Can you work these out from the drawing? Everything is in mm from the part's minimum corner. A direction names the side the tool comes from. Round coordinates to 2 decimals unless told otherwise and drop trailing zeros. Order: outer loops, then holes, each group sorted by start corner. A loop starts at its lowest first (then second) coordinate and runs counter-clockwise, first axis right, second up. Notation, with made-up numbers: (29.5, 46.25) -> (65.5, 46.25) arc R33 ccw to (65.5, 78.25) -> close; hole circle Ø7 at (33.5, 20). An arc over 180 degrees is marked (long way). One line per item, written item: value.
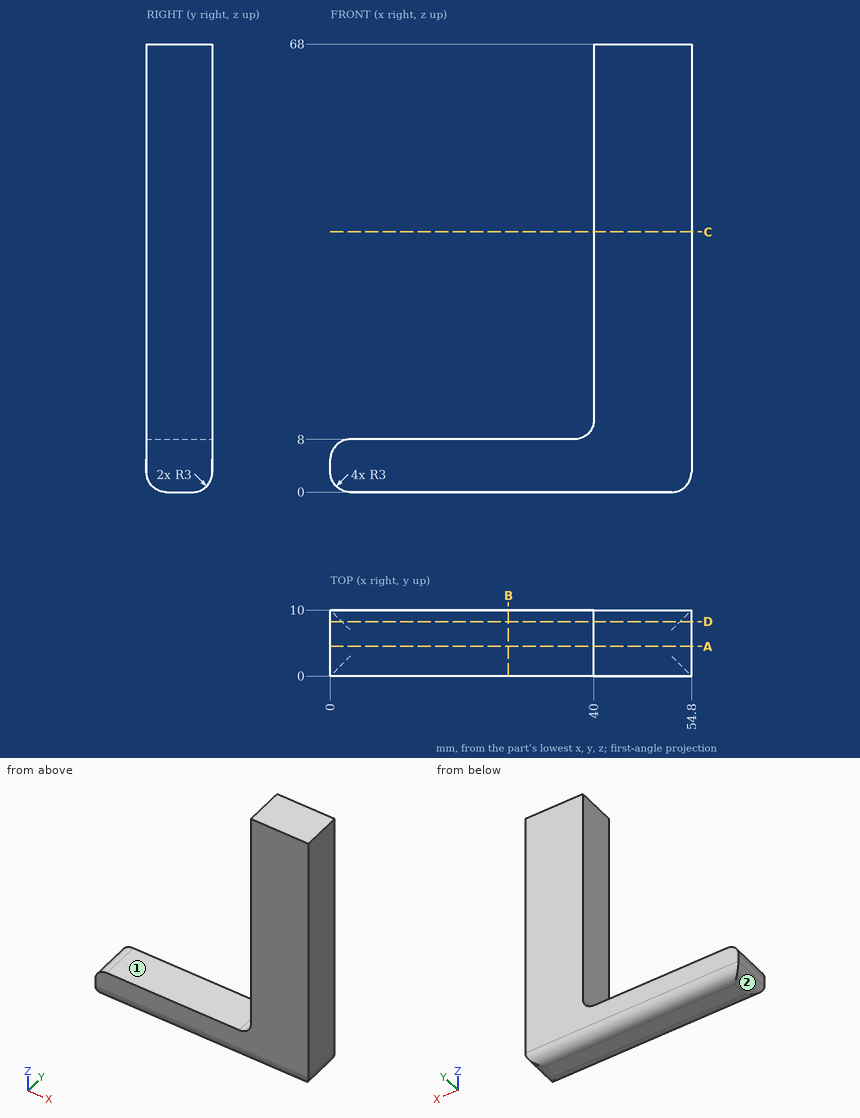
Q1. I want a section at A-A on y = 4.5. List the corners of the cut face in (x, z) for me.
Answers below:
outline: (0, 3) arc R3 ccw to (3, 0) -> (51.8, 0) arc R3 ccw to (54.8, 3) -> (54.8, 68) -> (40, 68) -> (40, 11) arc R3 cw to (37, 8) -> (3, 8) arc R3 ccw to (0, 5) -> close
Q2. Will these pins go through, and if not, where does the flat tip stop? pin 1 Ø6 at (x, y) = (31.5, 3.5) entering from +Z; pin 2 Ø1.5 at (y, z) = (3, 24.5) entering from -X; pin 3 Ø2 at (y, z) = (7, 8.5) entering from -X.
Answers below:
pin 1: z = 8
pin 2: x = 40
pin 3: x = 1.34
Q3. On a 3-axis mill with a long thin cutter (end or side, diameter ignored), from which of +Z, -Z, +X, -X, +Y, -Y can I reach the whole of each face in a straight line? I mean the marked faces 1 and 2. Say none if no direction works.
Answers below:
face 1: +Z, -X, +Y, -Y
face 2: -Z, -X, +Y, -Y
Q4. Please list where these lines run through material, in increasing order: line 1 along X through (y, z) = (4, 35); line 2 along Z through (x, y) = (52, 5.25); line 3 along Z through (x, y) = (35, 6.75).
Answers below:
line 1: 40 to 54.8
line 2: 0.01 to 68
line 3: 0 to 8
Q5. I want a section at B-B on x = 27. List the corners of the cut face in (y, z) for me, plus the area to 3 significant figures.
Answers below:
outline: (0, 3) arc R3 ccw to (3, 0) -> (7, 0) arc R3 ccw to (10, 3) -> (10, 8) -> (0, 8) -> close
area: 76.1 mm^2
Q6. I want a section at D-D on y = 8.25. List the corners of the cut face in (x, z) for me.
Answers below:
outline: (0, 3) arc R3 ccw to (1.75, 0.27) -> (53.05, 0.27) arc R3 ccw to (54.8, 3) -> (54.8, 68) -> (40, 68) -> (40, 11) arc R3 cw to (37, 8) -> (3, 8) arc R3 ccw to (0, 5) -> close
Q7. I want a section at C-C on z = 39.5. List the corners of the cut face in (x, y) for me, plus the area to 3 significant figures.
Answers below:
outline: (40, 0) -> (54.8, 0) -> (54.8, 10) -> (40, 10) -> close
area: 148 mm^2
